Here's how the part is built. I have some questions about the finished solid (model axes, mm). Face numbers are marked on the shaded views. Give positions to 0.01 mm unless a question says otherwise; leave off trailing zeros. Order: outer loops, then holes, each group sorted by start corner. A loop starts at its lowest first (then second) coordinate and runs counter-clockwise, first axis right, second up. Notation, with made-up numbers: (-27.5, 68) -> (-22.5, 68) arc R14 ccw to (-22.5, 89) -> close; hole circle Ø4 at (-27.75, 37.25). An arc over 180 degrees is marked (long way). Write each question's results on one line, items separated by ' | '. Start each with the question number.
Q1. Imagine slicing it at B-B, the plane x = 0. Please give me the cut outline in (y, z).
Q2. I need wall thicknesses on line 1 along Y through (x, z) = (0, -1.3); line 2 along X through (y, z) = (0, 5); line 3 along Z through (x, y) = (-15, 6). Which ranges of each line are inside material? Lowest first, please. Write a range as [from, to].
Q3. Imagine slicing it at C-C, the plane z = 1. Please give me the cut outline in (x, y), then the cut area to 3 significant figures.
Q4. Imagine slicing it at D-D, the plane x = 24.5. Please give me the cut outline in (y, z), then the cut area to 3 significant figures.
Q5. Imagine slicing it at A-A, the plane y = 0. Please give me the cut outline in (x, z), then the cut area to 3 significant figures.
Q6. Thinking about a two-plate mould opening in Y: for the marked faces 1, 2 and 3, which applies, pulls with the +Y half, pulls with the -Y half, needs draft (parallel to the pull), parting line crosses it, or undercut?
Q7. I'm going to push flat-ended pins straight in: pin 1 (0.6 mm diameter, centred on x = 0, y = -38.5, fed in from +Z); pin 2 (5 mm diameter, centred on x = -25.5, y = -18.5, fed in from +Z); pin 3 (6 mm diameter, centred on x = -16.5, z = 1, fed in from -Y); pin 4 (1.9 mm diameter, centred on x = 0, y = 0, fed in from -Z). Where does each tip first touch, or does it pass through?
```python
from build123d import *

# Parameters (mm, degrees)
SKETCH2_R           = 39.554
SKETCH2_R_2         = 38.354
BOSS_EXTRUDE1_DEPTH = 12.7
BOSS_EXTRUDE2_START = -2
SKETCH2_2_R         = 39.554
BOSS_EXTRUDE2_DEPTH = 2
SKETCH4_R           = 1.5875
CUT_EXTRUDE1_DEPTH  = 58.837080078
CUT_EXTRUDE3_REACH  = 59.361
SKETCH5_W           = 13.208
SKETCH5_H           = 10.16
FILLET1_R           = 2.54


with BuildPart() as part:
    # Sketch2 → Boss-Extrude1 (new body)
    with BuildSketch(Plane.XY):
        Circle(SKETCH2_R)
        Circle(SKETCH2_R_2, mode=Mode.SUBTRACT)
    extrude(amount=BOSS_EXTRUDE1_DEPTH)

    # Sketch2<2> → Boss-Extrude2 (add)
    with BuildSketch(Plane.XY.offset(BOSS_EXTRUDE2_START)):
        Circle(SKETCH2_2_R)
    extrude(amount=BOSS_EXTRUDE2_DEPTH)

    # Sketch4 → Cut-Extrude1 (cut, through all)
    with BuildSketch(Plane(origin=(0, 0, -2), x_dir=(-1, 0, 0), z_dir=(0, 0, -1))):
        Circle(SKETCH4_R)
    extrude(amount=-CUT_EXTRUDE1_DEPTH, mode=Mode.SUBTRACT)

    # Sketch5 → Cut-Extrude3 (cut, up to next)
    with BuildSketch(Plane(origin=(0, 0, 0), x_dir=(1, 0, 0), z_dir=(0, 1, 0)), mode=Mode.PRIVATE) as cut_extrude3_sk1:
        with Locations((0, -7.62)):
            Rectangle(SKETCH5_W, SKETCH5_H)
    cut_extrude3_tool1 = extrude(cut_extrude3_sk1.sketch, amount=-CUT_EXTRUDE3_REACH, mode=Mode.PRIVATE) & part.part
    add(cut_extrude3_tool1.solids().sort_by_distance((0, 0, 7.62))[0], mode=Mode.SUBTRACT)

    # Fillet1
    # the kernel refuses this fillet: 2.54 mm, written as the material it takes off along each edge
    with BuildSketch(Plane(origin=(-6.604, -37.781165943, 17.336288805), x_dir=(0, -1, 0), z_dir=(0, 0, -1))) as fillet1_piece_1:
        with BuildLine():
            CenterArc((2.114605309, 2.376349225), FILLET1_R, 192.685578689, 56.634940698)
            Line((-0.363392905, 1.818563559), (-0.41295287, 1.807407846))
            ThreePointArc((-0.41295287, 1.807407846), (-0.220518494, 0.901524198), (-0.050041279, -0.00874702))
            Line((-0.050041279, -0.00874702), (0, -0.0508))
            ThreePointArc((0, -0.0508), (0.608815096, -0.0508), (1.19969069, -0.047526985))
            Line((1.19969069, -0.047526985), (1.217630192, 0))
        make_face()
    extrude(amount=14.796288805, mode=Mode.SUBTRACT)
    with BuildSketch(Plane(origin=(6.604, -37.781165943, 17.336288805), x_dir=(0, -1, 0), z_dir=(0, 0, -1))) as fillet1_piece_2:
        with BuildLine():
            CenterArc((2.114605309, -2.376349225), FILLET1_R, 110.679480614, 56.634940698)
            Line((-0.363392905, -1.818563559), (-0.41295287, -1.807407846))
            ThreePointArc((-0.41295287, -1.807407846), (-0.220518494, -0.901524198), (-0.050041279, 0.00874702))
            Line((-0.050041279, 0.00874702), (0, 0.0508))
            ThreePointArc((0, 0.0508), (0.608815096, 0.0508), (1.19969069, 0.047526985))
            Line((1.19969069, 0.047526985), (1.217630192, 0))
        make_face()
    extrude(amount=14.796288805, mode=Mode.SUBTRACT)


solid = part.part
```
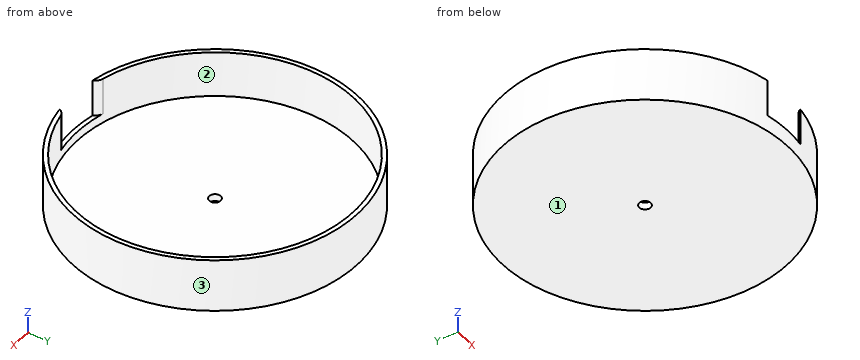
Geometry check:
1) outline: (-39.55, -2) -> (-1.59, -2) -> (-1.59, 0) -> (-38.35, 0) -> (-38.35, 2.54) -> (-39.55, 2.54) -> close; (1.59, -2) -> (39.55, -2) -> (39.55, 12.7) -> (38.35, 12.7) -> (38.35, 0) -> (1.59, 0) -> close
2) line 1: [-39.55, -1.59], [1.59, 39.55] | line 2: [-39.55, -38.35], [38.35, 39.55] | line 3: [-2, 0]
3) outline: circle Ø79.11 at (0, 0); hole circle Ø76.71 at (0, 0) | area: 294 mm²
4) outline: (-31.05, -2) -> (31.05, -2) -> (31.05, 12.7) -> (29.51, 12.7) -> (29.51, 0) -> (-29.51, 0) -> (-29.51, 12.7) -> (-31.05, 12.7) -> close | area: 163 mm²
5) outline: (-39.55, -2) -> (-1.59, -2) -> (-1.59, 0) -> (-38.35, 0) -> (-38.35, 12.7) -> (-39.55, 12.7) -> close; (1.59, -2) -> (39.55, -2) -> (39.55, 12.7) -> (38.35, 12.7) -> (38.35, 0) -> (1.59, 0) -> close | area: 182 mm²
6) face 1: needs draft | face 2: undercut | face 3: parting line crosses it
7) pin 1: z = 2.54 | pin 2: z = 0 | pin 3: y = -37.18 | pin 4: through
